Geometry: see drawing. Coordinates: mm, zero at the bounding-box minimum. Round coordinates to 2 decimals unless told otherwise and drop trailing zeros. Loops run counter-clockwise (first coordinate to the right, second up) from the corner with the lowest first, then second, coordinate; pieces in that order, holes last.
(1) Section C-C, the plane y = 1. Return the cut outline in (x, z).
(2) Section D-D, the plane x = 73. Return the cut outline in (y, z), plus the area to 3 significant figures.
(3) Section B-B, the plane z = 18. Return the cut outline in (x, y).
(4) First-contact query: pin 1 Ø6.5 at (x, z) = (73, 128) entering from -Y. Flat tip, straight axial feed; report the tip coordinate or a pass-through.
(5) Material intervals for probe 1 along X at (y, z) = (0.8, 73); probe 2 along Z at (x, y) = (128, 0.4), sorted ascending.
(6) Section A-A, the plane x = 128. Return the cut outline in (y, z).
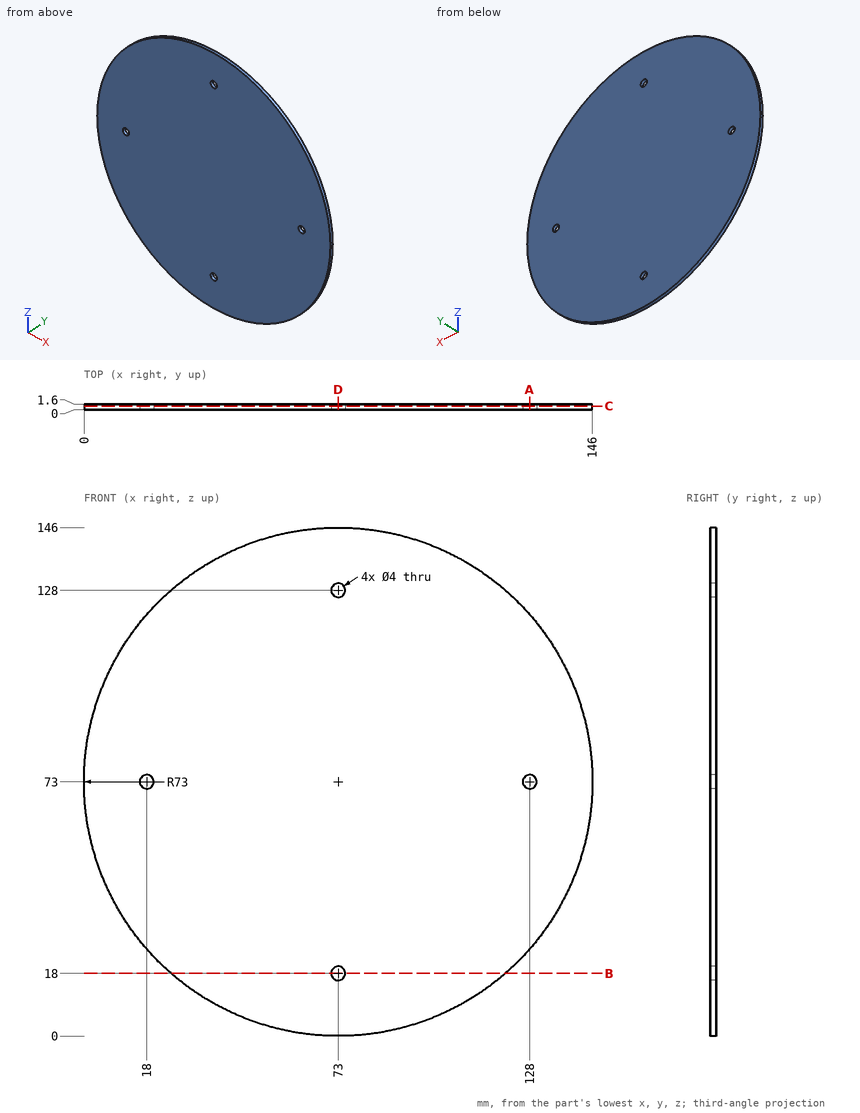
Output values:
1. outline: circle Ø146 at (73, 73); hole circle Ø4 at (18, 73); hole circle Ø4 at (73, 18); hole circle Ø4 at (73, 128); hole circle Ø4 at (128, 73)
2. outline: (0, 0) - (1.6, 0) - (1.6, 16) - (0, 16) - close; (0, 20) - (1.6, 20) - (1.6, 126) - (0, 126) - close; (0, 130) - (1.6, 130) - (1.6, 146) - (0, 146) - close
2. area: 221 mm2
3. outline: (25, 0) - (71, 0) - (71, 1.6) - (25, 1.6) - close; (75, 0) - (121, 0) - (121, 1.6) - (75, 1.6) - close
4. pin 1: stops at y = 0
5. probe 1: x = 0 to 16, 20 to 126, 130 to 146
5. probe 2: z = 25 to 71, 75 to 121
6. outline: (0, 25) - (1.6, 25) - (1.6, 71) - (0, 71) - close; (0, 75) - (1.6, 75) - (1.6, 121) - (0, 121) - close
